CAD build for the part. Positions are in the model's coordinates, mm. Face numbers are marked on the shaded views. Coordinates: 2 decimals unless noted, no trailing zeros. Order: outer loops, then holes, each group sorted by start corner. A loop starts at its lowest first (then second) coordinate and runs counter-clockwise, first axis right, second up. Notation, with made-up numbers: M 3,22.25 L 17,22.25 A19 cw 17,55.25 Z; hole C 8.5,3.25 d2. An arc over 180 degrees is marked long. Write item = value, one per line.
from build123d import *

# Parameters (mm, degrees)
SKETCH_1_R      = 10
SKETCH_1_R_2    = 1.5
EXTRUDE_1_DEPTH = 1.5
FILLET_1_R      = 0.3


with BuildPart() as part:
    # 草图1 → 凸台-拉伸1 (new body)
    with BuildSketch(Plane(origin=(0, 0, 0), x_dir=(1, 0, 0), z_dir=(0, 1, 0))):
        with Locations(Location((0, 0, 0), (0, 0, 270))):
            Circle(SKETCH_1_R)
        with Locations(Location((0, 7, 0), (0, 0, 270))):
            Circle(SKETCH_1_R_2, mode=Mode.SUBTRACT)
        with Locations(Location((0, -7, 0), (0, 0, 270))):
            Circle(SKETCH_1_R_2, mode=Mode.SUBTRACT)
    extrude(amount=EXTRUDE_1_DEPTH)

    # 圆角1
    fillet_1_edges = [part.edges().sort_by_distance(p)[0] for p in [
        (0, 0, -10),
        (0, 1.5, -10),
    ]]
    fillet(fillet_1_edges, radius=FILLET_1_R)


solid = part.part
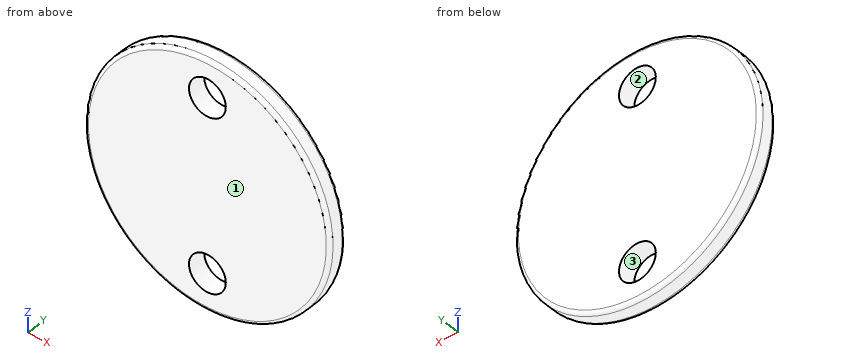
(1) Wall check: line 1 (X direction, y = 0.85, z = 0.25); line 2 (Z direction, x = 0.75, y = 0.25); line 3 (X direction, y = 0.9, z = -5.75). Give the ranges that are in metal, low to high. Write a range as from..to.
Evaluation:
line_1 = -10..10
line_2 = -9.97..-8.3, -5.7..5.7, 8.3..9.97
line_3 = -8.18..-0.83, 0.83..8.18
(2) Pin check, flat tip, straight feed: pin 1 Ø2.5 at (x, z) = (0, 7) entering from -Y. Stop position of the tip, or through.
Evaluation:
pin_1 = through
(3) Slice it at B-B, the plane x = -0.5. State how many separate pieces and enclosed holes the cut face has, then the cut area to 3 significant figures.
Evaluation:
separate_pieces = 3
enclosed_holes = 0
area = 21.4 mm²
(4) Slice it at A-A, the plane y = 0.9. Write the cut outline in (x, z), then the cut area to 3 significant figures.
Evaluation:
outline = C 0,0 d20; hole C 0,-7 d3; hole C 0,7 d3
area = 300 mm²
(5) Pull direction Z, two halves, no side cores. Call the marked faces 1, 2 and 3: +Z half, -Z half, draft (parallel to the pull), parting line (faces both ways), or undercut.
Evaluation:
face_1 = draft
face_2 = undercut
face_3 = undercut
